Geometry check sheet. Reference: the model listing, model coordinates, mm. Face numbers are marked on the shaded views. A direction names the side the tool comes from. Give positions to 0.01 mm unless a question says otherwise; leave off trailing zeros. Order: outer loops, then holes, each group sorted by start corner. A loop starts at its lowest first (then second) coordinate and runs counter-clockwise, first axis right, second up. Notation, with made-up numbers: M 11,-3.5 L 27,-3.5 A32 cw 27,23.5 Z; hole C 4.5,34 d7. An arc over 180 degrees is marked long. One line per question, with ' | ' between items. Start each with the question number.
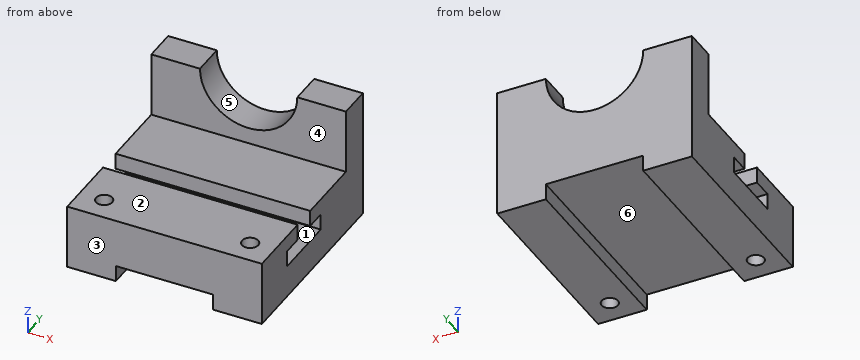
from build123d import *

# Parameters (mm, degrees)
F1_DEPTH = 152.4
F2_W     = 76.2
F2_H     = 12.7
F3_DEPTH = 152.4
F5_DEPTH = 171.70927
F7_R     = 6.35
F8_DEPTH = 152.4


with BuildPart() as f1:
    # F0 (on Right) → F1 (new body)
    with BuildSketch(Plane.YZ):
        Polygon((0, 50.8), (0, 0), (152.4, 0), (152.4, 101.6), (127, 101.6), (127, 50.8), (73.025, 50.8), (73.025, 38.1), (88.9, 38.1), (88.9, 25.4), (38.1, 25.4), (38.1, 38.1), (53.975, 38.1), (53.975, 50.8), align=None)
    extrude(amount=F1_DEPTH)

    # F2 (on Front) → F3 (cut)
    with BuildSketch(Plane.XZ):
        with Locations((76.2, 6.35)):
            Rectangle(F2_W, F2_H)
    extrude(amount=-F3_DEPTH, mode=Mode.SUBTRACT)

    # F4 (on Front) → F5 (cut)
    with BuildSketch(Plane.XZ):
        with BuildLine():
            ThreePointArc((38.1, 101.6), (76.2, 63.5), (114.3, 101.6))
            Line((114.3, 101.6), (38.1, 101.6))
        make_face()
        with BuildLine():
            Line((38.1, 101.6), (114.3, 101.6))
            ThreePointArc((114.3, 101.6), (76.2, 139.7), (38.1, 101.6))
        make_face()
    extrude(amount=-F5_DEPTH, mode=Mode.SUBTRACT)

    # F7 (on Top) → F8 (cut)
    with BuildSketch(Plane.XY):
        with Locations((19.05, 19.05)):
            Circle(F7_R)
        with Locations((133.35, 19.05)):
            Circle(F7_R)
    extrude(amount=F8_DEPTH, mode=Mode.SUBTRACT)


solid = f1.part
Item 1: Material ranges on line 1 along X through (y, z) = (19.05, 23); line 2 along X through (y, z) = (19.05, 11.5); line 3 along Y through (x, z) = (19.05, 28), recorded low to high.
Item 2: Set-up check for the marked faces 4, 5 and 6: record each of +Z, -Z, +X, -X, +Y, -Y from which the full face is reachable in a straight line by a thin tool's end or side.
Item 3: Cross-section at D-D, the plane y = 19.05. Record the cut outline in (x, z), plus the area to 3 significant figures.
Item 4: Cross-section at B-B, the plane z = 74.5. Record the cut outline in (x, y), plus the area to 3 significant figures.
Item 5: Depth check by flat-ended pin: pin 1 (12.5 mm diameter, centred on x = 47.5, y = 79.5, fed in from -Z); pin 2 (15 mm diameter, centred on x = 41, z = 74.5, fed in from -Y); pin 3 (15 mm diameter, centred on x = 93.5, y = 59.5, fed in from +Z). Enter the tip coordinate at first touch or a pass-through.
Item 6: Cross-section at C-C, the plane x = 133.35. Record the cut outline in (y, z) (3 decimals), plus the area to 3 significant figures.
Item 7: Mould release check, pull along Y, two halves, no side actions. Record for the marked faces 1, 2 and 3: released by +Y, released by -Y, zero draft, split by the parting line, or undercut.
Item 8: Cross-section at A-A, the plane y = 75.5. Record the cut outline in (x, z), plus the area to 3 significant figures.
Outcome:
1) line 1: x = 0 to 12.7, 25.4 to 127, 139.7 to 152.4 | line 2: x = 0 to 12.7, 25.4 to 38.1, 114.3 to 127, 139.7 to 152.4 | line 3: y = 0 to 12.7, 25.4 to 38.1, 88.9 to 152.4
2) face 4: +Z, +X, -X, -Y | face 5: +Z, +Y, -Y | face 6: -Z, +Y, -Y
3) outline: M 0,0 L 12.7,0 L 12.7,50.8 L 0,50.8 Z; M 25.4,0 L 38.1,0 L 38.1,12.7 L 114.3,12.7 L 114.3,0 L 127,0 L 127,50.8 L 25.4,50.8 Z; M 139.7,0 L 152.4,0 L 152.4,50.8 L 139.7,50.8 Z | area: 5,480 mm²
4) outline: M 0,127 L 49.42,127 L 49.42,152.4 L 0,152.4 Z; M 102.98,127 L 152.4,127 L 152.4,152.4 L 102.98,152.4 Z | area: 2,510 mm²
5) pin 1: stops at z = 12.7 | pin 2: stops at y = 127 | pin 3: stops at z = 50.8
6) outline: M 0,0 L 12.7,0 L 12.7,50.8 L 0,50.8 Z; M 25.4,0 L 152.4,0 L 152.4,101.6 L 127,101.6 L 127,50.8 L 73.025,50.8 L 73.025,38.1 L 88.9,38.1 L 88.9,25.4 L 38.1,25.4 L 38.1,38.1 L 53.975,38.1 L 53.975,50.8 L 25.4,50.8 Z | area: 7,500 mm²
7) face 1: undercut | face 2: zero draft | face 3: released by -Y
8) outline: M 0,0 L 38.1,0 L 38.1,12.7 L 114.3,12.7 L 114.3,0 L 152.4,0 L 152.4,25.4 L 0,25.4 Z; M 0,38.1 L 152.4,38.1 L 152.4,50.8 L 0,50.8 Z | area: 4,840 mm²
